from build123d import *

# Parameters (mm, degrees)
SKETCH1_W           = 200
SKETCH1_H           = 200
BOSS_EXTRUDE1_DEPTH = 200
SHELL1_T            = -4
CUT_EXTRUDE1_REACH  = 302
SKETCH2_R           = 1.5
SKETCH2_R_2         = 5


with BuildPart() as part:
    # Sketch1 → Boss-Extrude1 (new body)
    with BuildSketch(Plane(origin=(0, 0, 0), x_dir=(1, 0, 0), z_dir=(0, 1, 0))):
        Rectangle(SKETCH1_W, SKETCH1_H)
    extrude(amount=BOSS_EXTRUDE1_DEPTH)

    # Shell1
    shell1_openings = [part.faces().sort_by_distance(p)[0] for p in [
        (0, 200, 0),
    ]]
    offset(amount=SHELL1_T, openings=shell1_openings, kind=Kind.INTERSECTION)

    # Sketch2 → Cut-Extrude1 (cut, up to next)
    with BuildSketch(Plane.XY.offset(100), mode=Mode.PRIVATE) as cut_extrude1_sk1:
        with Locations((-12.5, 137.5)):
            Circle(SKETCH2_R)
    cut_extrude1_tool1 = extrude(cut_extrude1_sk1.sketch, amount=-CUT_EXTRUDE1_REACH, mode=Mode.PRIVATE) & part.part
    # Sketch2 → Cut-Extrude1 (cut, up to next)
    with BuildSketch(Plane.XY.offset(100), mode=Mode.PRIVATE) as cut_extrude1_sk2:
        with Locations((12.5, 137.5)):
            Circle(SKETCH2_R)
    cut_extrude1_tool2 = extrude(cut_extrude1_sk2.sketch, amount=-CUT_EXTRUDE1_REACH, mode=Mode.PRIVATE) & part.part
    # Sketch2 → Cut-Extrude1 (cut, up to next)
    with BuildSketch(Plane.XY.offset(100), mode=Mode.PRIVATE) as cut_extrude1_sk3:
        with Locations((12.5, 112.5)):
            Circle(SKETCH2_R)
    cut_extrude1_tool3 = extrude(cut_extrude1_sk3.sketch, amount=-CUT_EXTRUDE1_REACH, mode=Mode.PRIVATE) & part.part
    # Sketch2 → Cut-Extrude1 (cut, up to next)
    with BuildSketch(Plane.XY.offset(100), mode=Mode.PRIVATE) as cut_extrude1_sk4:
        with Locations((-12.5, 112.5)):
            Circle(SKETCH2_R)
    cut_extrude1_tool4 = extrude(cut_extrude1_sk4.sketch, amount=-CUT_EXTRUDE1_REACH, mode=Mode.PRIVATE) & part.part
    # Sketch2 → Cut-Extrude1 (cut, up to next)
    with BuildSketch(Plane.XY.offset(100), mode=Mode.PRIVATE) as cut_extrude1_sk5:
        with Locations((0, 95)):
            Circle(SKETCH2_R_2)
    cut_extrude1_tool5 = extrude(cut_extrude1_sk5.sketch, amount=-CUT_EXTRUDE1_REACH, mode=Mode.PRIVATE) & part.part
    add(cut_extrude1_tool1.solids().sort_by_distance((-12.5, 137.5, 100))[0], mode=Mode.SUBTRACT)
    add(cut_extrude1_tool2.solids().sort_by_distance((12.5, 137.5, 100))[0], mode=Mode.SUBTRACT)
    add(cut_extrude1_tool3.solids().sort_by_distance((12.5, 112.5, 100))[0], mode=Mode.SUBTRACT)
    add(cut_extrude1_tool4.solids().sort_by_distance((-12.5, 112.5, 100))[0], mode=Mode.SUBTRACT)
    add(cut_extrude1_tool5.solids().sort_by_distance((0, 95, 100))[0], mode=Mode.SUBTRACT)


solid = part.part
Design review of the part built by this model. Coordinates are the model's own, in mm. A direction names the side the tool comes from. Round coordinates to 2 decimals unless told otherwise and drop trailing zeros. Loops run counter-clockwise (first coordinate to the right, second up) from the corner with the lowest first, then second, coordinate; pieces in that order, holes last. Notation, with made-up numbers: (51, -28) - (82, -28) arc R35 ccw to (82, 6) - close; hole circle Ø3 at (37.5, 64.25). An arc over 180 degrees is marked (long way). One line per question, with ' | ' between items.
1. Draft analysis for pull direction Z (two halves, no side actions). For faces 1 (the face through (-100, 99, 1)), 2 (the face through (-1, 99, -100)), 3 (the face through (-1, 76, 100)), 4 (the face through (-1, 101, 96)), state which applies: released by +Z, released by -Z, zero draft, split by the parting line, or undercut.
Results are:
face 1: zero draft | face 2: released by -Z | face 3: released by +Z | face 4: undercut
2. We need section A-A, the plane y = 40.5. State the section outline as (x, z) points.
Results are:
outline: (-100, -100) - (100, -100) - (100, 100) - (-100, 100) - close; hole (-96, -96) - (96, -96) - (96, 96) - (-96, 96) - close
3. We need section C-C, the plane z = -1. State the section outline as (x, y) points.
Results are:
outline: (-100, 0) - (100, 0) - (100, 200) - (96, 200) - (96, 4) - (-96, 4) - (-96, 200) - (-100, 200) - close
4. We need section B-B, the plane x = -44.5. State the section outline as (y, z) points, and give its area (3 significant figures).
Results are:
outline: (0, -100) - (200, -100) - (200, -96) - (4, -96) - (4, 96) - (200, 96) - (200, 100) - (0, 100) - close | area: 2,370 mm²
5. For L1, parallel to Y at x = 12.5, z = 96.95; L2, parallel to X at y = 112.5, z = 98.6; L3, parallel to X at y = 144, z = -24.5, list the stretches that pass through material, from the lowest coordinate up. Write a range as [from, to].
Results are:
L1: y = [0, 111], [114, 136], [139, 200] | L2: x = [-100, -14], [-11, 11], [14, 100] | L3: x = [-100, -96], [96, 100]
6. Clearance check with flat-ended pins moving along their axes: P1, Ø12, axis at x = 53, z = 39, coming from the +Y side; P2, Ø6, axis at x = 0, y = 95, coming from the +Z side. State where each tip first meets the part, or that it passes through.
Results are:
P1: stops at y = 4 | P2: stops at z = -96
7. For faces 5 (the face through (-97, 200, -45)), 6 (the face through (96, 101, 1)), 7 (the face through (-1.08, 90.12, 98.03)), list the 3-axis set-ups (+Z, -Z, +X, -X, +Y, -Y) from which the entire face can be reached by the end or side of a thin tool; tool diameter is ignored.
Results are:
face 5: +Z, -Z, +X, -X, +Y | face 6: +Y | face 7: +Z
